from build123d import *

# Parameters (mm, degrees)
BASE_FLANGE1_DEPTH  = 2.5
SKETCH8_W           = 0.4
SKETCH8_H           = 3.67
BOSS_EXTRUDE1_DEPTH = 4.5
SKETCH9_W           = 3.4
SKETCH9_H           = 1
CUT_EXTRUDE1_DEPTH  = 11.945052861
FILLET1_RADIUS      = 1.335
FILLET1_LENGTH      = 0.4


# Sheet-metal steps are written as plain solids
with BuildPart() as part:
    # Sketch3 → Base-Flange1 (new body)
    with BuildSketch(Plane.XY):
        with BuildLine():
            Line((0.71, -1.835), (0.71, 1.835))
            ThreePointArc((0.71, 1.835), (0, 2.545), (-0.71, 1.835))
            Line((-0.71, 1.835), (-0.71, -2.335))
            ThreePointArc((-0.71, -2.335), (-0.993802137, -2.877286979), (-1.601136872, -2.953203645))
            Line((-1.601136872, -2.953203645), (-6.752833912, -1.027063048))
            Line((-6.752833912, -1.027063048), (-6.61275096, -0.652394172))
            Line((-6.61275096, -0.652394172), (-1.461053919, -2.578534769))
            ThreePointArc((-1.461053919, -2.578534769), (-1.221800842, -2.548628204), (-1.11, -2.335))
            Line((-1.11, -2.335), (-1.11, 1.835))
            ThreePointArc((-1.11, 1.835), (0, 2.945), (1.11, 1.835))
            Line((1.11, 1.835), (1.11, -1.835))
            Line((1.11, -1.835), (0.71, -1.835))
        make_face()
    extrude(amount=BASE_FLANGE1_DEPTH)

    # Sketch8 → Boss-Extrude1 (add)
    with BuildSketch(Plane.XY.offset(2.5)):
        with Locations((0.91, 0)):
            Rectangle(SKETCH8_W, SKETCH8_H)
    extrude(amount=BOSS_EXTRUDE1_DEPTH)

    # Sketch9 → Cut-Extrude1 (cut, through all)
    with BuildSketch(Plane(origin=(1.11, 0, 0), x_dir=(0, 0, -1), z_dir=(1, 0, 0))):
        with Locations((-5.3, -1.335)):
            Rectangle(SKETCH9_W, SKETCH9_H)
    extrude(amount=-CUT_EXTRUDE1_DEPTH, mode=Mode.SUBTRACT)

    # Fillet1: full round fillet: the end face becomes a half cylinder, R = half its width
    fillet1_face = Plane((0.91, 0.5, 7), x_dir=(-1, 0, 0), z_dir=(0, 0, 1))  # on the end face: x along it, z out of the body
    fillet1_slab = fillet1_face.offset(-FILLET1_RADIUS / 2) * Box(FILLET1_LENGTH, 2 * FILLET1_RADIUS, FILLET1_RADIUS, mode=Mode.PRIVATE)  # the body's end, R deep
    fillet1_round = Plane((0.91, 0.5, 5.665), x_dir=(0, 0, 1), z_dir=(-1, 0, 0)) * Cylinder(FILLET1_RADIUS, FILLET1_LENGTH, mode=Mode.PRIVATE)  # its axis R under the face
    add(fillet1_slab - fillet1_round, mode=Mode.SUBTRACT)


solid = part.part
Read the model definition and answer for the solid it produces. Units are mm, in the model's axes. A direction names the side the tool comes from. Round coordinates to 2 decimals unless told otherwise and drop trailing zeros. Write each loop counter-clockwise with the first axis right and the second up, starting at its lowest first coordinate (ties: lowest second). Pieces come first, ordered by that corner, then holes. Notation, with made-up numbers: (-36, -11.75) - (-27, -11.75) arc R19 cw to (-27, 25.25) - close; hole circle Ø11 at (51.25, -10). An arc over 180 degrees is marked (long way). Use a Markdown table: item, result.
(1) The part is cut by section A-A (y = 0.5). Write down the section's boundary in (x, z), then the cut area to 3 significant figures.
Reported:
| item | result |
|---|---|
| outline | (-1.11, 0) - (-0.71, 0) - (-0.71, 2.5) - (-1.11, 2.5) - close; (0.71, 0) - (1.11, 0) - (1.11, 7) - (0.71, 7) - close |
| area | 3.80 mm2 |
(2) Straight lines are drawn through the part: line 1 along X through (y, z) = (0.3, 1.25); line 2 along X through (y, z) = (-0.1, 6.75); line 3 along Z through (x, y) = (-1, 0.6). For each, find the intervals that lie inside material, in ascending order. Write a range as [from, to].
Reported:
| item | result |
|---|---|
| line 1 | [-1.11, -0.71], [0.71, 1.11] |
| line 2 | [0.71, 1.11] |
| line 3 | [0, 2.5] |
(3) The mould has two halves that part along X. Classify faces 1 (the cylindrical face through (0.016, 2.545, 1.232)), 2 (the flat face through (-4.141, -2.004, 1.232)), 3 (the flat face through (-4.073, -1.602, 1.232)), 4 (the cylindrical face through (-0.024, 2.945, 1.232)): released by +X, released by -X, zero draft, split by the parting line, or undercut.
Reported:
| item | result |
|---|---|
| face 1 | undercut |
| face 2 | released by -X |
| face 3 | undercut |
| face 4 | split by the parting line |
(4) The part is cut by section C-C (y = 1.1). Write down the section's boundary in (x, z).
Reported:
| item | result |
|---|---|
| outline | (-1.11, 0) - (-0.71, 0) - (-0.71, 2.5) - (-1.11, 2.5) - close; (0.71, 0) - (1.11, 0) - (1.11, 6.86) - (0.71, 6.86) - close |
(5) Which of the six approach directions +Z, -Z, +X, -X, +Y, -Y give full straight-line access (tool end or side, diameter ignored) to faces 5 (the flat face through (-1.11, 0, 1)), 6 (the flat face through (1.11, 0, 3)), 7 (the flat face through (0.71, 0, 3))?
Reported:
| item | result |
|---|---|
| face 5 | +Z, -Z, +Y |
| face 6 | +Z, -Z, +X, +Y, -Y |
| face 7 | +Z, -Z, -Y |
(6) The part is cut by section D-D (x = 0). Write down the section's boundary in (y, z) (3 decimals), then the cut area to 4 significant figures.
Reported:
| item | result |
|---|---|
| outline | (2.545, 0) - (2.945, 0) - (2.945, 2.5) - (2.545, 2.5) - close |
| area | 1.000 mm2 |
(7) The part is cut by section B-B (z = 2.25). Write down the section's boundary in (x, y) (3 decimals), then the cut area to 3 significant figures.
Reported:
| item | result |
|---|---|
| outline | (-6.753, -1.027) - (-1.601, -2.953) arc R0.66 ccw to (-0.71, -2.335) - (-0.71, 1.835) arc R0.71 cw to (0.71, 1.835) - (0.71, -1.835) - (1.11, -1.835) - (1.11, 1.835) arc R1.11 ccw to (-1.11, 1.835) - (-1.11, -2.335) arc R0.26 cw to (-1.461, -2.579) - (-6.613, -0.652) - close |
| area | 6.83 mm2 |
(8) Each of these flat-tipped pins is pushed along its axis until it touches: pin 1 Ø1.2 at (y, z) = (0.5, 1) entering from -X; pin 2 Ø1.5 at (x, z) = (-4, 1.5) entering from +Y; pin 3 Ø1.8 at (y, z) = (-1, 4) entering from -X. Where does it stop, or does it pass through?
Reported:
| item | result |
|---|---|
| pin 1 | x = -1.11 |
| pin 2 | y = -1.35 |
| pin 3 | x = 0.71 |
